```python
from build123d import *

# Parameters (mm, degrees)
SKETCH_R        = 9.25
PAD_DEPTH       = 4.5
SKETCH001_R     = 5
PAD001_DEPTH    = 8
SKETCH002_R     = 4
PAD002_DEPTH    = 17.5
SKETCH003_W     = 3.5
SKETCH003_H     = 10
POCKET_DEPTH    = 11
CHAMFER_SIZE    = 0.5
CHAMFER001_SIZE = 1


with BuildPart() as part:
    # Sketch → Pad (new body)
    with BuildSketch(Plane.XY):
        Circle(SKETCH_R)
    extrude(amount=PAD_DEPTH)

    # Sketch001 (on Face3 of Pad) → Pad001 (join)
    with BuildSketch(Plane.XY.offset(4.5)):
        Circle(SKETCH001_R)
    extrude(amount=PAD001_DEPTH)

    # Sketch002 (on Face5 of Pad001) → Pad002 (join)
    with BuildSketch(Plane.XY.offset(12.5)):
        Circle(SKETCH002_R)
    extrude(amount=PAD002_DEPTH)

    # Sketch003 (on Face2 of Pad002) → Pocket (cut)
    with BuildSketch(Plane(origin=(0, 0, 0), x_dir=(1, 0, 0), z_dir=(0, 0, -1))):
        Rectangle(SKETCH003_W, SKETCH003_H)
    extrude(amount=-POCKET_DEPTH, mode=Mode.SUBTRACT)

    # Chamfer
    chamfer_edges = [part.edges().sort_by_distance(p)[0] for p in [
        (-4, 0, 30),
        (-5, 0, 12.5),
        (-9.25, 0, 0),
    ]]
    chamfer(chamfer_edges, length=CHAMFER_SIZE)

    # Chamfer001
    chamfer001_edges = [part.edges().sort_by_distance(p)[0] for p in [
        (0, -5, 0),
        (1.75, 0, 0),
        (0, 5, 0),
        (-1.75, 0, 0),
    ]]
    chamfer(chamfer001_edges, length=CHAMFER001_SIZE)


solid = part.part
```
Geometry: final body of the model. Coordinates: model frame, mm. A direction names the side the tool comes from. Round coordinates to 2 decimals unless told otherwise and drop trailing zeros. Order: outer loops, then holes, each group sorted by start corner. A loop starts at its lowest first (then second) coordinate and runs counter-clockwise, first axis right, second up. Notation, with made-up numbers: M -17,56 L 30,56 A16 cw 30,80 Z; hole C 7,-23 d11. An arc over 180 degrees is marked long. Use one line per item in the form item = value. Start each with the question number.
Q1. Cut plane B-B (y = 0). Return loops of the section in (x, z).
Q2. Mould query, pull axis Y, two halves, no side actions, for faces 1 (the face through (4.619, -1.915, 8.198)), 2 (the face through (4, 0, 0)), 3 (the face through (0, -5, 3)). Classes: +Y half, -Y half, draft (parallel to the pull), parting line (faces both ways), or undercut.
Q3. Cut plane C-C (z = 21.5). Return loops of the section in (x, y).
Q4. Pin query (flat end, axial travel): pin 1 Ø2 at (y, z) = (2.5, 21) entering from -X; pin 2 Ø8 at (x, z) = (2.5, 21.5) entering from -Y; pin 3 Ø3 at (y, z) = (-3, 24.5) entering from +X. Return the tip coordinate at first contact, or that it passes through.
Q5. Cut plane A-A (x = 0). Return loops of the section in (y, z), and give its area (4 significant figures).
Q6. Access query for faces 4 (the face through (0, 0, 11)), 5 (the face through (0, 5.5, 0.5)), 6 (the face through (-0.867, -3.905, 20.881)). Directions: +Z, -Z, +X, -X, +Y, -Y. A direction counts if a zero-diameter tool reaches every point of the face in a straight line with its end or side. Return the directions, or none.
Q7. Material intervals for line 1 (Z direction, x = 3, y = 7.5); line 2 (X direction, y = 2.5, z = 2); line 3 (Z direction, x = -2.25, y = -5.25), sorted ascending. Write a range as [from, to].
Q8. Cut plane D-D (z = 8.75). Return loops of the section in (x, y).
Geometry results:
q1.outline = M -9.25,0.5 L -8.75,0 L -2.75,0 L -1.75,1 L -1.75,11 L 1.75,11 L 1.75,1 L 2.75,0 L 8.75,0 L 9.25,0.5 L 9.25,4.5 L 5,4.5 L 5,12 L 4.5,12.5 L 4,12.5 L 4,29.5 L 3.5,30 L -3.5,30 L -4,29.5 L -4,12.5 L -4.5,12.5 L -5,12 L -5,4.5 L -9.25,4.5 Z
q2.face_1 = parting line
q2.face_2 = draft
q2.face_3 = undercut
q3.outline = C 0,0 d8
q4.pin_1 = -3.71
q4.pin_2 = -4
q4.pin_3 = 3.71
q5.outline = M -9.25,0.5 L -8.75,0 L -6,0 L -5,1 L -5,4.5 L -9.25,4.5 Z; M -5,11 L 5,11 L 5,12 L 4.5,12.5 L 4,12.5 L 4,29.5 L 3.5,30 L -3.5,30 L -4,29.5 L -4,12.5 L -4.5,12.5 L -5,12 Z; M 5,1 L 6,0 L 8.75,0 L 9.25,0.5 L 9.25,4.5 L 5,4.5 Z
q5.area = 191.5 mm^2
q6.face_4 = -Z, +Y, -Y
q6.face_5 = -Z
q6.face_6 = +Z
q7.line_1 = [0, 4.5]
q7.line_2 = [-8.91, -1.75], [1.75, 8.91]
q7.line_3 = [0.5, 4.5]
q8.outline = M -1.75,-4.68 L -1.75,4.68 A5 ccw Z; M 1.75,-4.68 A5 ccw 1.75,4.68 Z
